```python
from build123d import *

# Parameters (mm, degrees)
BOSS_EXTRUDE1_DEPTH = 1.27
SKETCH2_R           = 1.143
CUT_EXTRUDE2_DEPTH  = 2.54
SKETCH3_R           = 2.54
SKETCH3_R_2         = 1.143
CUT_EXTRUDE3_DEPTH  = 2.54
SKETCH19_W          = 30.913141625
SKETCH19_H          = 1.27
BOSS_EXTRUDE2_DEPTH = 3.81
SKETCH20_W          = 33.557604238
SKETCH20_H          = 1.27
BOSS_EXTRUDE3_DEPTH = 3.81
SKETCH21_W          = 109.982
SKETCH21_H          = 6.204110365
BOSS_EXTRUDE4_DEPTH = 2.54
SKETCH22_R          = 1.143
CUT_EXTRUDE6_DEPTH  = 2.54


with BuildPart() as part:
    # Sketch1 → Boss-Extrude1 (new body)
    with BuildSketch(Plane(origin=(0, 0, 0), x_dir=(1, 0, 0), z_dir=(0, 1, 0))):
        Polygon((49.53, -54.991), (49.53, -11.176), (67.31, -11.176), (67.31, 11.176), (49.53, 11.176), (49.53, 54.991), (-49.53, 54.991), (-49.53, 21.433395762), (-46.907297859, 21.433395762), (-46.907297859, -24.077858375), (-49.53, -24.077858375), (-49.53, -54.991), align=None)
    extrude(amount=BOSS_EXTRUDE1_DEPTH)

    # Sketch2 → Cut-Extrude2 (cut)
    with BuildSketch(Plane(origin=(0, 1.27, 0), x_dir=(1, 0, 0), z_dir=(0, 1, 0))):
        with Locations(Location((63.345949026, 0, 0), (0, 0, 270))):
            Circle(SKETCH2_R)
    extrude(amount=-CUT_EXTRUDE2_DEPTH, mode=Mode.SUBTRACT)

    # Sketch3 → Cut-Extrude3 (cut)
    with BuildSketch(Plane(origin=(0, 1.27, 0), x_dir=(1, 0, 0), z_dir=(0, 1, 0))):
        with Locations(Location((-6.5275, 11.696076054, 0), (0, 0, 270))):
            Circle(SKETCH3_R)
        with Locations(Location((9.3475, 11.696076054, 0), (0, 0, 270))):
            Circle(SKETCH3_R)
        with Locations(Location((-6.5275, -7.461873946, 0), (0, 0, 270))):
            Circle(SKETCH3_R_2)
        with Locations(Location((9.3475, -7.461873946, 0), (0, 0, 270))):
            Circle(SKETCH3_R_2)
    extrude(amount=-CUT_EXTRUDE3_DEPTH, mode=Mode.SUBTRACT)

    # Sketch19 → Boss-Extrude2 (add)
    with BuildSketch(Plane.ZY.offset(49.53)):
        with Locations((39.534429188, 0.635)):
            Rectangle(SKETCH19_W, SKETCH19_H)
    extrude(amount=BOSS_EXTRUDE2_DEPTH)

    # Sketch20 → Boss-Extrude3 (add)
    with BuildSketch(Plane.ZY.offset(49.53)):
        with Locations((-38.212197881, 0.635)):
            Rectangle(SKETCH20_W, SKETCH20_H)
    extrude(amount=BOSS_EXTRUDE3_DEPTH)

    # Sketch21 → Boss-Extrude4 (add)
    with BuildSketch(Plane.ZY.offset(53.34)):
        with Locations((0, -1.832055183)):
            Rectangle(SKETCH21_W, SKETCH21_H)
    extrude(amount=BOSS_EXTRUDE4_DEPTH)

    # Sketch22 → Cut-Extrude6 (cut)
    with BuildSketch(Plane.ZY.offset(55.88)):
        with Locations((-0.192674888, -1.428814134)):
            Circle(SKETCH22_R)
    extrude(amount=-CUT_EXTRUDE6_DEPTH, mode=Mode.SUBTRACT)


solid = part.part
```
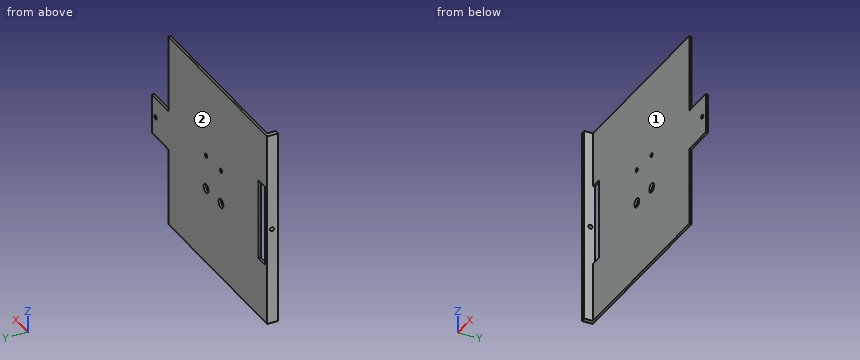
Input: part model. Units: mm. Frame: model coordinates. Face numbers are marked on the shaded views. A direction names the side the tool comes from. Give positions to 0.01 mm unless a question says otherwise; leave off trailing zeros. Loops run counter-clockwise (first coordinate to the right, second up) from the corner with the lowest first, then second, coordinate; pieces in that order, holes last. Notation, with made-up numbers: M -18,20.5 L 25,20.5 A14 ccw 25,26.5 Z; hole C 3,-10 d6. An arc over 180 degrees is marked long. Answer as CSV lines item,"result". Start each with the question number.
1. Section D-D on x = 17.5. Return loops of the section in (y, z).
2. Section B-B on z = -47. Return loops of the section in (x, y).
3. Reachability of the marked faces 1 and 2 from +Z, -Z, +X, -X, +Y, -Y: full face, straight path, thin tool, end or side. Return the list, or none.
4. Section A-A on z = -4. Return loops of the section in (x, y), plus the area to 3 significant figures.
5. Line query: L1, parallel to X at y = 0.7, z = 0; L2, parallel to X at y = 0.5, z = -10; L3, parallel to X at y = -2.5, z = -40. Output: solid intervals per line, ascending.
6. Pin query (flat end, axial travel): P1, Ø8, axis at x = -13.5, z = -8.5, coming from the -Y side; P2, Ø0.6, axis at x = 58.5, y = 1, coming from the -Z side; P3, Ø1.4, axis at x = 9.35, z = 7.46, coming from the -Y side; P4, Ø3, axis at y = -3.5, z = -10.5, coming from the +X side. Return the tip coordinate at first contact, or that it passes through.
7. Section C-C on x = 54.5. Return loops of the section in (y, z).
Computed values:
1,outline,"M 0,-54.99 L 1.27,-54.99 L 1.27,54.99 L 0,54.99 Z"
2,outline,"M -55.88,-4.93 L -53.34,-4.93 L -53.34,0 L 49.53,0 L 49.53,1.27 L -55.88,1.27 Z"
3,face 1,"+Z, -Z, +X, -Y"
3,face 2,"+Z, -Z, +X, -X, +Y"
4,outline,"M -55.88,-4.93 L -53.34,-4.93 L -53.34,1.27 L -55.88,1.27 Z; M -46.91,0 L 67.31,0 L 67.31,1.27 L -46.91,1.27 Z"
4,area,"161 mm²"
5,L1,"x = -55.88 to -53.34, -46.91 to 62.2, 64.49 to 67.31"
5,L2,"x = -55.88 to -53.34, -46.91 to -8.42, -4.64 to 7.46, 11.24 to 67.31"
5,L3,"x = -55.88 to -53.34"
6,P1,"stops at y = 0"
6,P2,"stops at z = -11.18"
6,P3,"passes through"
6,P4,"stops at x = -53.34"
7,outline,"M 0,-11.18 L 1.27,-11.18 L 1.27,11.18 L 0,11.18 Z"
